Read the model definition and answer for the solid it produces. Units are mm, in the model's axes. A direction names the side the tool comes from. Round coordinates to 2 decimals unless told otherwise and drop trailing zeros. Order: outer loops, then holes, each group sorted by start corner. A loop starts at its lowest first (then second) coordinate and runs counter-clockwise, first axis right, second up.
from build123d import *

# Parameters (mm, degrees)
EXTRUDE_3_8_DEPTH = 9.525
SKETCH2_R         = 2
M4_DRILL_DEPTH    = 8
SKETCH3_R         = 2
M4_DRILL2_DEPTH   = 8


with BuildPart() as part:
    # Sketch1 → 3/8 (new body)
    with BuildSketch(Plane.XY):
        Polygon((0, 0), (18, 0), (18, 8), (8, 8), (8, 18), (0, 18), align=None)
    extrude(amount=EXTRUDE_3_8_DEPTH)

    # Sketch2 → M4_DRILL (cut)
    with BuildSketch(Plane.ZY):
        with Locations(Location((4.7625, 14, 0), (0, 0, 270))):
            Circle(SKETCH2_R)
    extrude(amount=-M4_DRILL_DEPTH, mode=Mode.SUBTRACT)

    # Sketch3 → M4_DRILL2 (cut)
    with BuildSketch(Plane(origin=(0, 0, 0), x_dir=(-1, 0, 0), z_dir=(0, -1, 0))):
        with Locations(Location((-14, -4.7625, 0), (0, 0, 180))):
            Circle(SKETCH3_R)
    extrude(amount=-M4_DRILL2_DEPTH, mode=Mode.SUBTRACT)


solid = part.part
Q1. A cutting plane is placed at A-A, the plane y = 14. Give the vertices of the cut face in (x, z) (1 decimal).
Outcome:
outline: (0, 0) - (8, 0) - (8, 2.8) - (0, 2.8) - close; (0, 6.8) - (8, 6.8) - (8, 9.5) - (0, 9.5) - close
Q2. Straight lines are drawn through the part: probe 1 along Z at (x, y) = (3.25, 14) (1 decimal); probe 2 along Y at (x, z) = (9.75, 8). For each, find the intervals that lie inside material, in ascending order.
Outcome:
probe 1: z = 0 to 2.8, 6.8 to 9.5
probe 2: y = 0 to 8
Q3. For a pull along Z with two mould halves and no side action, classify faces 3 (the face through (4, 18, 5)), 4 (the face through (3.944, 14.26, 6.745)), 5 (the face through (7, 7, 9.525)) as released by +Z, released by -Z, zero draft, split by the parting line, or undercut.
Outcome:
face 3: zero draft
face 4: undercut
face 5: released by +Z
Q4. Flat-ended cylindrical pins translate along their axes: pin 1 (4 mm diameter, centred on x = 12.5, z = 4.5, fed in from +Y); pin 2 (3 mm diameter, centred on x = 14, z = 4.76, fed in from +Y). Find the tip coordinate at first contact, or state that the pin passes through.
Outcome:
pin 1: stops at y = 8
pin 2: passes through
Q5. A cutting plane is placed at C-C, the plane z = 6.5. Give the vertices of the cut face in (x, y).
Outcome:
outline: (0, 0) - (13.01, 0) - (13.01, 8) - (8, 8) - (8, 13.01) - (0, 13.01) - close; (0, 14.99) - (8, 14.99) - (8, 18) - (0, 18) - close; (14.99, 0) - (18, 0) - (18, 8) - (14.99, 8) - close
Q6. For faces 1 (the face through (9, 0, 5)), 2 (the face through (8, 11.8, 4.7)), determine the directions among +Z, -Z, +X, -X, +Y, -Y from which every point of the face is accessible in a straight line to the end or side of a thin tool.
Outcome:
face 1: +Z, -Z, +X, -X, -Y
face 2: +Z, -Z, +X, +Y
Q7. A cutting plane is placed at D-D, the plane z = 1.75. Give the vertices of the cut face in (x, y), plus the area to 3 significant figures.
Outcome:
outline: (0, 0) - (18, 0) - (18, 8) - (8, 8) - (8, 18) - (0, 18) - close
area: 224 mm2
